from build123d import *

# Parameters (mm, degrees)
SKETCH_W     = 20
SKETCH_H     = 20
PAD_DEPTH    = 2
PAD001_DEPTH = 2.5
CHAMFER_SIZE = 1
FILLET_R     = 1


with BuildPart() as part:
    # Sketch → Pad (new body)
    with BuildSketch(Plane.XY):
        Rectangle(SKETCH_W, SKETCH_H)
    extrude(amount=PAD_DEPTH)

    # Sketch001 → Pad001 (join, symmetric)
    with BuildSketch(Plane.XZ):
        with BuildLine():
            ThreePointArc((8.921584, 2), (7.836918, 7.610703), (3.592669, 11.437298))
            ThreePointArc((3.592669, 11.437298), (0.950236, 8.958289), (4.545503, 8.508849))
            ThreePointArc((6.898889, 2), (6.582918, 5.565633), (4.545503, 8.508849))
            Line((6.898889, 2), (8.921584, 2))
        make_face()
        with BuildLine():
            Line((-8.921584, 2), (-6.898889, 2))
            ThreePointArc((-4.545503, 8.508849), (-6.582918, 5.565633), (-6.898889, 2))
            ThreePointArc((-4.545503, 8.508849), (-0.950236, 8.958289), (-3.592669, 11.437298))
            ThreePointArc((-3.592669, 11.437298), (-7.836918, 7.610703), (-8.921584, 2))
        make_face()
    extrude(amount=PAD001_DEPTH, both=True)

    # Chamfer
    chamfer_edges = [part.edges().sort_by_distance(p)[0] for p in [
        (-6.898889, 0, 2),
        (8.921584, 0, 2),
        (-8.921584, 0, 2),
        (6.898889, 0, 2),
    ]]
    chamfer(chamfer_edges, length=CHAMFER_SIZE)

    # Fillet
    fillet_edges = [part.edges().sort_by_distance(p)[0] for p in [
        (10, -10, 1),
        (10, 10, 1),
        (-10, -10, 1),
        (-10, 10, 1),
    ]]
    fillet(fillet_edges, radius=FILLET_R)


solid = part.part
Build history of the part. All positions in model axes, mm. A direction names the side the tool comes from. Coordinates: 2 decimals unless noted, no trailing zeros. Order: outer loops, then holes, each group sorted by start corner. A loop starts at its lowest first (then second) coordinate and runs counter-clockwise, first axis right, second up. Notation, with made-up numbers: (31.25, 46) - (85.25, 46) arc R13 cw to (85.25, 70) - close; hole circle Ø10 at (28.5, 10.25). An arc over 180 degrees is marked (long way). Write item = value, one per line. Start each with the question number.
1) Saw through at A-A on z = 5.5. Write the cut outline in (x, y), then the cut area to 3 significant figures.
2) Saw through at D-D on x = -0.25. Write the cut outline in (y, z).
3) Wall check: line 1 along X through (y, z) = (-0.75, 8.25); line 2 along Z through (x, y) = (3.75, -8); line 3 along Z through (x, y) = (-2.5, 2.25). Give the ranges that are in metal, low to high. Write a range as from..to.
4) Saw through at B-B on x = -4.25. Write the cut outline in (y, z), then the cut area to 3 significant figures.
5) Saw through at C-C on y = -0.75. Write the cut outline in (x, z), then the cut area to 3 significant figures.
6) Two-plate mould, pull along X, no slides. Class faces 1 (the face through (6.414, 0.035, 5.99)), 2 (the face through (-10, 0, 1)), 3 (the face through (9.699, 9.715, 1.014)): pulls with the +X half, pulls with the -X half, needs draft (parallel to the pull), parting line crosses it, or undercut.
7) 3-axis set-ups, long thin cutter, end or side, ignore diameter. For faces 4 (the face through (0, 10, 1)), 5 (the face through (-9.699, -9.715, 1.014)), 6 (the face through (6, 2.5, 8)), 7 (the face through (-6, -2.5, 8)), 8 (the face through (-6.456, 0.035, 2.505)): which of +Z, -Z, +X, -X, +Y, -Y reach the whole face in a straight line?
8) Flat gauge pins, fed straight in: pin 1 Ø2 at (x, y) = (-6.5, 4.5) entering from +Z; pin 2 Ø4.5 at (x, z) = (-4.5, 7.5) entering from -Y. Where does each tip first touch, or does it go through?
From the geometry:
q1.outline = (-8.7, -2.5) - (-6.61, -2.5) - (-6.61, 2.5) - (-8.7, 2.5) - close; (6.61, -2.5) - (8.7, -2.5) - (8.7, 2.5) - (6.61, 2.5) - close
q1.area = 20.9 mm^2
q2.outline = (-10, 0) - (10, 0) - (10, 2) - (-10, 2) - close
q3.line_1 = -7.44..-4.83, -4.35..-1.36, 1.36..4.35, 4.83..7.44
q3.line_2 = 0..2
q3.line_3 = 0..2, 7.61..11.55
q4.outline = (-10, 0) - (10, 0) - (10, 2) - (-10, 2) - close; (-2.5, 8.14) - (2.5, 8.14) - (2.5, 11.12) - (-2.5, 11.12) - close
q4.area = 54.9 mm^2
q5.outline = (-10, 0) - (10, 0) - (10, 2) - (9.92, 2) - (9, 3) arc R9 ccw to (3.59, 11.44) arc R2 ccw (long way) to (4.55, 8.51) arc R7 cw to (7, 3) - (5.9, 2) - (-5.9, 2) - (-7, 3) arc R7 cw to (-4.55, 8.51) arc R2 ccw (long way) to (-3.59, 11.44) arc R9 ccw to (-9, 3) - (-9.92, 2) - (-10, 2) - close
q5.area = 102 mm^2
q6.face_1 = undercut
q6.face_2 = pulls with the -X half
q6.face_3 = pulls with the +X half
q7.face_4 = +Z, -Z, +X, -X, +Y
q7.face_5 = +Z, -Z, -X, -Y
q7.face_6 = +Z, +X, -X, +Y
q7.face_7 = +Z, +X, -X, -Y
q7.face_8 = +Y, -Y
q8.pin_1 = 2
q8.pin_2 = -2.5
